from build123d import *

# Parameters (mm, degrees)
F0_W     = 42.037
F0_H     = 320.04
F1_DEPTH = 762


with BuildPart() as f1:
    # F0 (on Front) → F1 (new body)
    with BuildSketch(Plane.XZ):
        Polygon((-209.2325, 160.02), (-21.0185, 160.02), (21.0185, 160.02), (209.2325, 160.02), (209.2325, 227.584), (-209.2325, 227.584), align=None)
        Rectangle(F0_W, F0_H)
        Polygon((21.0185, -160.02), (-21.0185, -160.02), (-209.2325, -160.02), (-209.2325, -227.584), (209.2325, -227.584), (209.2325, -160.02), align=None)
    extrude(amount=F1_DEPTH)


solid = f1.part
The model under review builds one solid part; all positions refer to its coordinate system, in mm. A direction names the side the tool comes from. Round coordinates to 2 decimals unless told otherwise and drop trailing zeros. Loops run counter-clockwise (first coordinate to the right, second up) from the corner with the lowest first, then second, coordinate; pieces in that order, holes last. Notation, with made-up numbers: M 45.5,79 L 99.5,79 A22 cw 99.5,94 Z; hole C 86.5,-5 d4. An arc over 180 degrees is marked long. Answer as a JSON object with one key per item and string values.
Item 1: Tool access review of faces 1 (the face through (-114, -376, -160.02)), 2 (the face through (209.232, -376, -194)), 3 (the face through (116, -376, -160.02)): name each direction out of +Z, -Z, +X, -X, +Y, -Y from which nothing blocks a thin tool from reaching the whole face with its end or side.
Check sheet entries:
{"face 1": "-X, +Y, -Y", "face 2": "+Z, -Z, +X, +Y, -Y", "face 3": "+X, +Y, -Y"}
Item 2: The part is to be moulded in two halves that separate along Z. For faces 4 (the face through (-3, -376, -227.584)), 5 (the face through (-209.232, -376, 194)), 6 (the face through (-21.018, -376, -2)), 7 (the face through (3, -376, 227.584)), say which applies: +Z half, -Z half, draft (parallel to the pull), parting line (faces both ways), or undercut.
Check sheet entries:
{"face 4": "-Z half", "face 5": "draft", "face 6": "undercut", "face 7": "+Z half"}
Item 3: We need section C-C, the plane z = -75. State the section outline as (x, y) points, and give its area (3 significant figures).
Check sheet entries:
{"outline": "M -21.02,-762 L 21.02,-762 L 21.02,0 L -21.02,0 Z", "area": "32,000 mm2"}
Item 4: Clearance check with flat-ended pins moving along their axes: P1, Ø1.5, axis at y = -487, z = 85.5, coming from the -X side; P2, Ø2, axis at y = -617.5, z = -64, coming from the +X side. State where each tip first meets the part, or that it passes through.
Check sheet entries:
{"P1": "x = -21.02", "P2": "x = 21.02"}
Item 5: For line 1 along Z through (x, y) = (36.5, -693); line 2 along X through (y, z) = (-307, 102), list the stretches that pass through material, from the lowest coordinate up.
Check sheet entries:
{"line 1": "-227.58 to -160.02, 160.02 to 227.58", "line 2": "-21.02 to 21.02"}
Item 6: We need section A-A, the plane x = 99.5. State the section outline as (y, z) points.
Check sheet entries:
{"outline": "M -762,-227.58 L 0,-227.58 L 0,-160.02 L -762,-160.02 Z; M -762,160.02 L 0,160.02 L 0,227.58 L -762,227.58 Z"}
Item 7: We need section B-B, the plane y = -701. State the section outline as (x, z) points.
Check sheet entries:
{"outline": "M -209.23,-227.58 L 209.23,-227.58 L 209.23,-160.02 L 21.02,-160.02 L 21.02,160.02 L 209.23,160.02 L 209.23,227.58 L -209.23,227.58 L -209.23,160.02 L -21.02,160.02 L -21.02,-160.02 L -209.23,-160.02 Z"}
